Work out the finished part from the listing and answer in its coordinate system (mm). Round coordinates to 2 decimals unless told otherwise and drop trailing zeros. Write each loop counter-clockwise with the first axis right and the second up, starting at its lowest first coordinate (ties: lowest second). Pieces come first, ordered by that corner, then holes.
1. Flat-ended cylindrical pins translate along their axes: pin 1 Ø2 at (x, z) = (-8, 6.5) entering from -Y; pin 2 Ø1 at (y, z) = (12, 3) entering from -X; pin 3 Ø1 at (y, z) = (-11, 2) entering from -X. Find the tip coordinate at first contact, or state that the pin passes through.
2. Straight lines are drawn through the part: probe 1 along Z at (x, y) = (5, 11); probe 2 along Y at (x, z) = (-1.5, 7.5); probe 3 along Z at (x, y) = (0, 9.5). For each, find the intervals that lie inside material, in ascending order.
3. Find section B-B (x = 9.5). Write down the section's boundary in (y, z), and give its area (3 significant figures).
4. Find section A-A (z = 4). Write down the section's boundary in (x, y).
```python
from build123d import *

# Parameters (mm, degrees)
F1_DEPTH = 8.128
F2_R     = 5.08
F3_R     = 5.08


with BuildPart() as f1:
    # F0 (on Top) → F1 (new body)
    with BuildSketch(Plane.XY):
        Polygon((11.867368, -20.554884), (11.867368, 20.554884), (-23.734735, 0), align=None)
    extrude(amount=F1_DEPTH)

    # F2
    f2_edges = [f1.edges().sort_by_distance(p)[0] for p in [
        (11.867368, -20.554884, 4.064),
        (-23.734735, 0, 4.064),
        (11.867368, 20.554884, 4.064),
    ]]
    fillet(f2_edges, radius=F2_R)

    # F3
    f3_edges = [f1.edges().sort_by_distance(p)[0] for p in [
        (11.867368, 0, 8.128),
    ]]
    fillet(f3_edges, radius=F3_R)


solid = f1.part
```
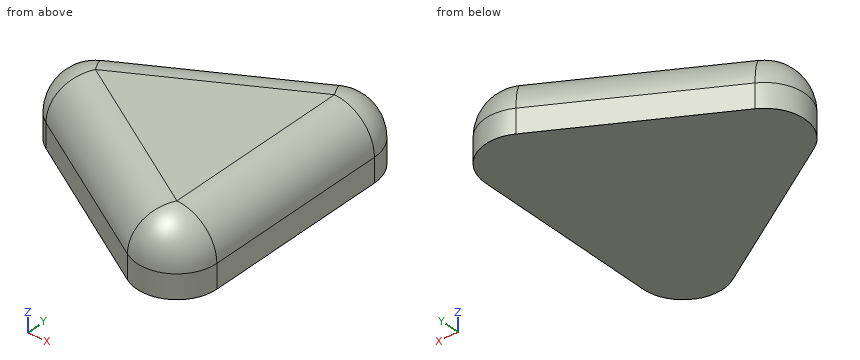
Worked answers:
1. pin 1: stops at y = -8.57
1. pin 2: stops at x = -3.82
1. pin 3: stops at x = -5.55
2. probe 1: z = 0 to 8.12
2. probe 2: y = -9.8 to 9.8
2. probe 3: z = 0 to 7.92
3. outline: (-16.05, 0) - (16.05, 0) - (16.05, 3.05) arc R4.3 ccw to (11.76, 7.34) - (-11.76, 7.34) arc R4.3 ccw to (-16.05, 3.05) - close
3. area: 228 mm2
4. outline: (-16.07, -4.32) - (4.29, -16.08) arc R4.99 ccw to (11.78, -11.76) - (11.78, 11.76) arc R4.99 ccw to (4.29, 16.08) - (-16.07, 4.32) arc R4.99 ccw to start
